from build123d import *

# Parameters (mm, degrees)
SKETCH_R        = 35.5
PAD_DEPTH       = 30
FILLET_R        = 2.5
FILLET001_R     = 2.5
SKETCH001_R     = 24
POCKET_DEPTH    = 20
SKETCH002_R     = 8.25
PAD001_DEPTH    = 16
POCKET001_DEPTH = 3
SKETCH004_R     = 1.5
POCKET002_DEPTH = 25


with BuildPart() as part:
    # Sketch → Pad (new body)
    with BuildSketch(Plane.YZ):
        with Locations((-2.086276, 2.086154)):
            Circle(SKETCH_R)
    extrude(amount=PAD_DEPTH)

    # Fillet
    fillet_edges = [part.edges().sort_by_distance(p)[0] for p in [
        (30, -37.586276, 2.086154),
    ]]
    fillet(fillet_edges, radius=FILLET_R)

    # Fillet001
    fillet001_edges = [part.edges().sort_by_distance(p)[0] for p in [
        (0, -37.586276, 2.086154),
    ]]
    fillet(fillet001_edges, radius=FILLET001_R)

    # Sketch001 (on Face3 of Pad) → Pocket (cut)
    with BuildSketch(Plane.YZ.offset(30)):
        with Locations((-2.490074, 1.413427)):
            Circle(SKETCH001_R)
    extrude(amount=-POCKET_DEPTH, mode=Mode.SUBTRACT)

    # Sketch002 (on Face7 of Pocket) → Pad001 (join)
    with BuildSketch(Plane.YZ.offset(10)):
        with Locations((-1.106776, 1.902246)):
            Circle(SKETCH002_R)
    extrude(amount=PAD001_DEPTH)

    # Sketch003 (on Face9 of Pad001) → Pocket001 (cut)
    with BuildSketch(Plane.YZ.offset(26)):
        Polygon((4.852949, 4.988847), (-1.209229, 8.488847), (-7.271407, 4.988847), (-7.271407, -2.011153), (-1.209229, -5.511153), (4.852949, -2.011153), align=None)
    extrude(amount=-POCKET001_DEPTH, mode=Mode.SUBTRACT)

    # Sketch004 (on Face16 of Pocket001) → Pocket002 (cut)
    with BuildSketch(Plane.YZ.offset(23)):
        with Locations((-1.040093, 1.343548)):
            Circle(SKETCH004_R)
    extrude(amount=-POCKET002_DEPTH, mode=Mode.SUBTRACT)


solid = part.part
Check sheet for the modelled part. Datum: model origin and axes. Units: mm. A direction names the side the tool comes from. Coordinates: 2 decimals unless noted, no trailing zeros. Write each loop counter-clockwise with the first axis right and the second up, starting at its lowest first coordinate (ties: lowest second). Pieces come first, ordered by that corner, then holes. Notation, with made-up numbers: M -4,-28 L 19,-28 A17 ccw 19,1 Z; hole C 18,8 d3. An arc over 180 degrees is marked long. Answer as CSV lines item,"result".
Q1. Set-up check for faces 4 (the face through (24.52, -4.2, 6.76)), 5 (the face through (11.66, -1.24, 2.83)): record each of +Z, -Z, +X, -X, +Y, -Y from which the full face is reachable in a straight line by a thin tool's end or side.
Check result:
face 4,"+X"
face 5,"+X, -X"
Q2. Cross-section at A-A (x = 21.5). Record the boundary of the cut face in (y, z), then the cut area to 3 significant figures.
Check result:
outline,"C -2.09,2.09 d71; C -1.11,1.9 d16.5; hole C -2.49,1.41 d48; hole C -1.04,1.34 d3"
area,"2,360 mm^2"
Q3. Material ranges on probe 1 along Y at (x, z) = (19.25, 1); probe 2 along X at (y, z) = (6, -4); probe 3 along Y at (x, z) = (25.5, -1.5), recorded low to high. Write a range as from..to.
Check result:
probe 1,"-37.57..-26.49, -9.31..-2.5, 0.42..7.09, 21.51..33.4"
probe 2,"0..10"
probe 3,"-37.4..-26.31, -8.62..-7.27, 4.85..6.41, 21.33..33.23"
Q4. Cross-section at B-B (x = 4.5). Record the boundary of the cut face in (y, z).
Check result:
outline,"C -2.09,2.09 d71; hole C -1.04,1.34 d3"
Q5. Mould release check, pull along Z, two halves, no side actions. Record for faces 1 (the face through (30, 5, 25)), 2 (the face through (14.82, 17, 32.02)), 3 (the face through (25, 4.853, 1)): released by +Z, released by -Z, zero draft, split by the parting line, or undercut.
Check result:
face 1,"zero draft"
face 2,"split by the parting line"
face 3,"undercut"
Q6. Go/stop test with flat-tipped pins: pin 1 (10 mm diameter, centred on x = 12, y = -4.5, fed in from +Z); pin 2 (3 mm diameter, centred on x = 25, z = 10, fed in from -Y); pin 3 (4 mm diameter, centred on x = 27, y = 23, fed in from +Z); pin 4 (3.5 mm diameter, centred on x = 24.5, z = 1.5, fed in from -Y). Record where each tip stops, or that it passes through.
Check result:
pin 1,"z = 37.59"
pin 2,"y = -37"
pin 3,"z = 29.05"
pin 4,"y = -37.59"
